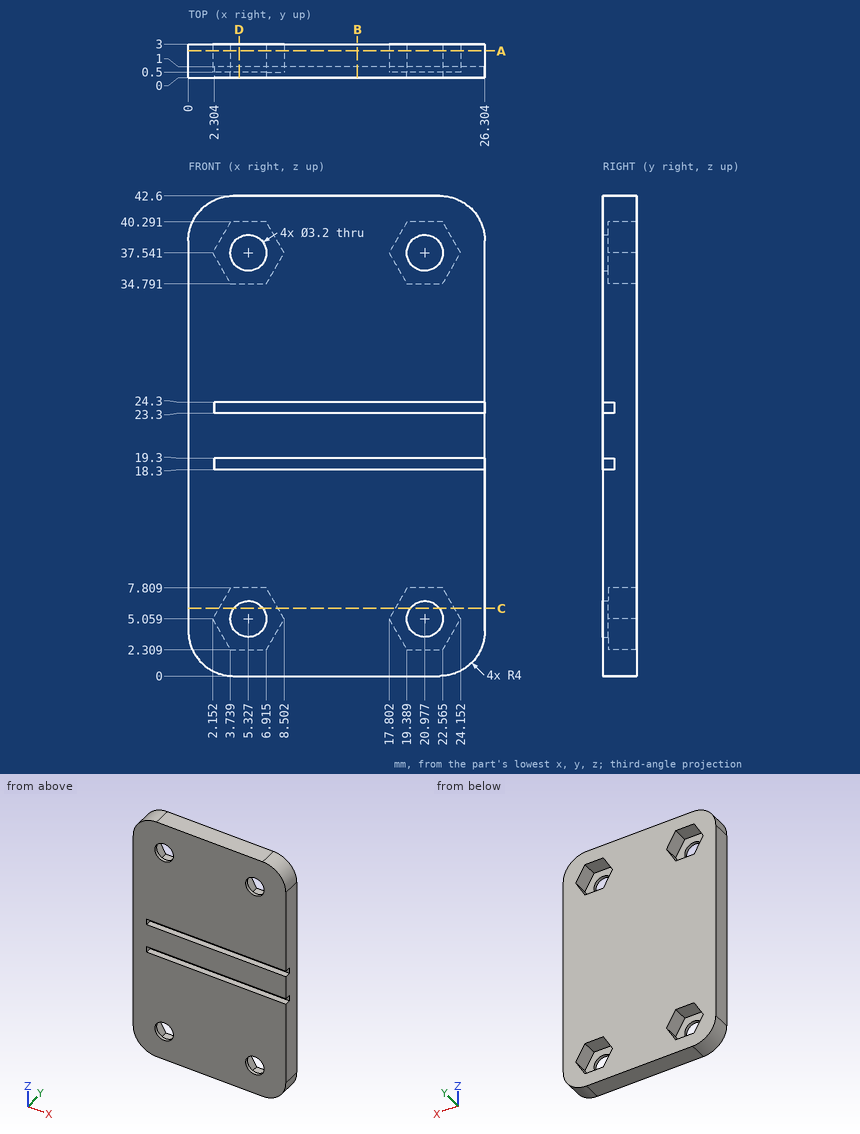
Geometry: see drawing. Coordinates: mm, zero at the bounding-box minimum. Coordinates: 2 decimals unless noted, no trailing zeros. Loops run counter-clockwise (first coordinate to the right, second up) from the corner with the lowest first, then second, coordinate; pieces in that order, holes last.
Q1. Cut plane A-A (y = 2.4). Give the number of separate pieces and of enclosed holes in the cut face, then the cut area to 3 significant figures.
Q2. Cut plane D-D (x = 4.5). Output: boundary loops of the cut face in (y, z).
Q3. Material intervals for line 1 (Z direction, x = 14.25, y = 0.6); line 2 (Z direction, x = 3.75, y = 1.6); line 3 (Z direction, x = 20.25, y = 0.7), sorted ascending.
Q4. Cut plane B-B (x = 15). Output: boundary loops of the cut face in (y, z).
Q5. Cut plane C-C (z = 6). Output: boundary loops of the cut face in (x, y) (1 decimal).
Q6. Contact query for a flat-ended pin moving along its axis: pin 1 (10 mm diameter, centred on x = 16, z = 18, fed in from -Y). Output: stop coordinate, or through.
Working result:
1. separate pieces: 1
1. enclosed holes: 4
1. area: 1,000 mm2
2. outline: (0, 0) - (3, 0) - (3, 2.31) - (0.5, 2.31) - (0.5, 3.69) - (0, 3.69) - close; (0, 6.43) - (0.5, 6.43) - (0.5, 7.81) - (3, 7.81) - (3, 34.79) - (0.5, 34.79) - (0.5, 36.17) - (0, 36.17) - (0, 24.3) - (1, 24.3) - (1, 23.3) - (0, 23.3) - (0, 19.3) - (1, 19.3) - (1, 18.3) - (0, 18.3) - close; (0, 38.91) - (0.5, 38.91) - (0.5, 40.29) - (3, 40.29) - (3, 42.6) - (0, 42.6) - close
3. line 1: z = 0 to 18.3, 19.3 to 23.3, 24.3 to 42.6
3. line 2: z = 0.01 to 2.31, 7.81 to 34.79, 40.29 to 42.59
3. line 3: z = 0 to 2.31, 7.81 to 18.3, 19.3 to 23.3, 24.3 to 34.79, 40.29 to 42.6
4. outline: (0, 0) - (3, 0) - (3, 42.6) - (0, 42.6) - (0, 24.3) - (1, 24.3) - (1, 23.3) - (0, 23.3) - (0, 19.3) - (1, 19.3) - (1, 18.3) - (0, 18.3) - close
5. outline: (0, 0) - (4, 0) - (4, 0.5) - (2.7, 0.5) - (2.7, 3) - (0, 3) - close; (6.6, 0) - (19.7, 0) - (19.7, 0.5) - (18.3, 0.5) - (18.3, 3) - (8, 3) - (8, 0.5) - (6.6, 0.5) - close; (22.3, 0) - (26.3, 0) - (26.3, 3) - (23.6, 3) - (23.6, 0.5) - (22.3, 0.5) - close
6. pin 1: stops at y = 0
